from build123d import *

# Parameters (mm, degrees)
BOSS_EXTRUDE6_DEPTH      = 22.6
BOSS_EXTRUDE6_DEPTH_BACK = 22.6
SKETCH9_R                = 1.5
BOSS_EXTRUDE7_START      = -22.6
BOSS_EXTRUDE7_OUTLINE_R  = 2.5
BOSS_EXTRUDE7_DEPTH      = 45.2
CUT_EXTRUDE1_DEPTH       = 21.2
CUT_EXTRUDE1_DEPTH_BACK  = 21.2
SKETCH9_30_R             = 1.5
BOSS_EXTRUDE8_DEPTH      = 22.6
BOSS_EXTRUDE8_DEPTH_BACK = 22.6
SKETCH9_31_R             = 1.5
FILLET1_R                = 4
CHAMFER1_SIZE            = 2
CHAMFER2_SIZE            = 10
SKETCH11_R               = 2.5
CUT_EXTRUDE5_DEPTH       = 4


# Read off the part's stored shape, not the designer's step: Boss-Extrude7
with BuildPart() as part:
    # Sketch9 → Boss-Extrude6 (new, two sides: drawn at the far end of the back side and taken through both)
    with BuildSketch(Plane.XY.offset(-BOSS_EXTRUDE6_DEPTH_BACK)):
        Polygon((10.55, -1.2), (30.962513099, -1.2), (30.962513099, 6.2), (25.90954056, 6.2), (25.90954056, 8.2), (25.90954056, 18), (9.45, 18), (7.014466094, 15.564466094), (7.014466094, 11.55), (10.55, 8.014466094), align=None)
        with Locations((15.35, 2.8)):
            Circle(SKETCH9_R, mode=Mode.SUBTRACT)
    extrude(amount=BOSS_EXTRUDE6_DEPTH + BOSS_EXTRUDE6_DEPTH_BACK)

    # Boss-Extrude7 outline → Boss-Extrude7 (add)
    with BuildSketch(Plane.XY.offset(BOSS_EXTRUDE7_START)):
        with BuildLine():
            Line((38.90954056, 18), (25.90954056, 18))
            Line((25.90954056, 18), (25.90954056, 16))
            Line((25.90954056, 16), (38.90954056, 16))
            ThreePointArc((38.90954056, 16), (67.193811807, 4.284271247), (78.90954056, -24))
            Line((78.90954056, -24), (78.90954056, -78))
            ThreePointArc((78.90954056, -78), (71.880103308, -94.970562748), (54.90954056, -102))
            Line((54.90954056, -102), (54.709540559, -102))
            ThreePointArc((54.709540559, -102), (37.738977811, -94.970562748), (30.709540559, -78))
            Line((30.709540559, -78), (30.709540559, -24.386722193))
            ThreePointArc((30.709540559, -24.386722193), (37.738977811, -7.416159445), (54.709540559, -0.386722193))
            Line((54.709540559, -0.386722193), (57.736465726, -0.386722193))
            ThreePointArc((57.736465726, -0.386722193), (61.526284336, -3.986931746), (64.638517317, -8.186722193))
            Line((64.638517317, -8.186722193), (54.709540559, -8.186722193))
            ThreePointArc((54.709540559, -8.186722193), (43.254410704, -12.931592338), (38.509540559, -24.386722193))
            Line((38.509540559, -24.386722193), (38.509540559, -78))
            ThreePointArc((38.509540559, -78), (43.254410704, -89.455129855), (54.709540559, -94.2))
            Line((54.709540559, -94.2), (54.90954056, -94.2))
            ThreePointArc((54.90954056, -94.2), (66.364670415, -89.455129855), (71.10954056, -78))
            Line((71.10954056, -78), (71.10954056, -24))
            ThreePointArc((71.10954056, -24), (61.678378914, -1.231161646), (38.90954056, 8.2))
            Line((38.90954056, 8.2), (25.90954056, 8.2))
            Line((25.90954056, 8.2), (25.90954056, 6.2))
            Line((25.90954056, 6.2), (30.962513099, 6.2))
            Line((30.962513099, 6.2), (30.962513099, -13.8))
            ThreePointArc((30.962513099, -13.8), (29.279020372, -18.974823911), (28.709540559, -24.386722193))
            Line((28.709540559, -24.386722193), (28.709540559, -78))
            ThreePointArc((28.709540559, -78), (36.324764249, -96.384776311), (54.709540559, -104))
            Line((54.709540559, -104), (54.90954056, -104))
            ThreePointArc((54.90954056, -104), (73.29431687, -96.384776311), (80.90954056, -78))
            Line((80.90954056, -78), (80.90954056, -24))
            ThreePointArc((80.90954056, -24), (68.608025369, 5.69848481), (38.90954056, 18))
        make_face()
        with BuildLine():
            Line((40.509540559, -78), (40.509540559, -52.193361097))
            Line((40.509540559, -52.193361097), (48.38692427, -52.193361097))
            ThreePointArc((48.38692427, -52.193361097), (50.213346482, -55.789555174), (53.809540559, -57.615977386))
            Line((53.809540559, -57.615977386), (53.809540559, -92.171450173))
            ThreePointArc((53.809540559, -92.171450173), (44.355314369, -87.717509969), (40.509540559, -78))
        make_face(mode=Mode.SUBTRACT)
        with BuildLine():
            Line((61.232156849, -52.193361097), (69.10954056, -52.193361097))
            Line((69.10954056, -52.193361097), (69.10954056, -78))
            ThreePointArc((69.10954056, -78), (65.26376675, -87.717509969), (55.80954056, -92.171450173))
            Line((55.80954056, -92.171450173), (55.809540559, -57.615977386))
            ThreePointArc((55.809540559, -57.615977386), (59.405734637, -55.789555174), (61.232156849, -52.193361097))
        make_face(mode=Mode.SUBTRACT)
        with Locations((54.809540559, -51.193361097)):
            Circle(BOSS_EXTRUDE7_OUTLINE_R, mode=Mode.SUBTRACT)
        with BuildLine():
            Line((48.38692427, -50.193361097), (40.509540559, -50.193361097))
            Line((40.509540559, -50.193361097), (40.509540559, -24.386722193))
            ThreePointArc((40.509540559, -24.386722193), (44.321085429, -14.705813145), (53.709540559, -10.221977225))
            Line((53.709540559, -10.221977225), (53.709540559, -44.787114146))
            ThreePointArc((53.709540559, -44.787114146), (50.177660219, -46.633132538), (48.38692427, -50.193361097))
        make_face(mode=Mode.SUBTRACT)
        with BuildLine():
            ThreePointArc((38.90954056, 6.2), (47.231770136, 5.030681957), (54.909540559, 1.613277807))
            Line((54.909540559, 1.613277807), (54.709540559, 1.613277807))
            ThreePointArc((54.709540559, 1.613277807), (43.121398237, -1.111951356), (33.962513099, -8.716340846))
            Line((33.962513099, -8.716340846), (33.962513099, 6.2))
            Line((33.962513099, 6.2), (38.90954056, 6.2))
        make_face(mode=Mode.SUBTRACT)
        with BuildLine():
            Line((55.709540559, -10.186722193), (65.765328692, -10.186722193))
            ThreePointArc((65.765328692, -10.186722193), (68.261583092, -16.89383372), (69.10954056, -24))
            Line((69.10954056, -24), (69.10954056, -50.193361097))
            Line((69.10954056, -50.193361097), (61.232156849, -50.193361097))
            ThreePointArc((61.232156849, -50.193361097), (59.369856551, -46.561566838), (55.709540559, -44.755970321))
            Line((55.709540559, -44.755970321), (55.709540559, -10.186722193))
        make_face(mode=Mode.SUBTRACT)
    extrude(amount=BOSS_EXTRUDE7_DEPTH)

    # Sketch9<30> → Cut-Extrude1 (cut, two sides: drawn at the far end of the back side and taken through both)
    # profile 1 of 2: a face of its own
    with BuildSketch(Plane.XY.offset(-CUT_EXTRUDE1_DEPTH_BACK)):
        Polygon((19.104002376, 5), (16.104002376, 5), (10.55, 4), (10.55, -1.2), (19.35, -1.2), (19.35, 5.043376018), align=None)
        with Locations((15.35, 2.8)):
            Circle(SKETCH9_30_R, mode=Mode.SUBTRACT)
    # profile 2 of 2: a face of its own
    with BuildSketch(Plane.XY.offset(-CUT_EXTRUDE1_DEPTH_BACK)):
        Polygon((10.55, 5.097056275), (16.104002376, 7), (19.104002376, 7), (25.90954056, 8.2), (25.90954056, 16), (16.104002376, 16), (7.014466094, 14.164466094), (7.014466094, 11.55), (10.55, 8.014466094), align=None)
    extrude(amount=CUT_EXTRUDE1_DEPTH + CUT_EXTRUDE1_DEPTH_BACK, mode=Mode.SUBTRACT)

    # Sketch9<31> → Boss-Extrude8 (add, two sides: drawn at the far end of the back side and taken through both)
    # profile 1 of 2: a face of its own
    with BuildSketch(Plane.XY.offset(-BOSS_EXTRUDE8_DEPTH_BACK)):
        with BuildLine():
            ThreePointArc((38.90954056, 18), (56.770808698, 14.012828104), (71.240841297, 2.808338118))
            Line((71.240841297, 2.808338118), (71.240841297, 8))
            Line((71.240841297, 8), (71.240841297, 18))
            Line((71.240841297, 18), (38.90954056, 18))
        make_face()
        with Locations((66.240841297, 13)):
            Circle(SKETCH9_31_R, mode=Mode.SUBTRACT)
    # profile 2 of 2: a face of its own
    with BuildSketch(Plane.XY.offset(-BOSS_EXTRUDE8_DEPTH_BACK)):
        with BuildLine():
            Line((54.709540559, -104), (54.90954056, -104))
            ThreePointArc((54.90954056, -104), (57.370590519, -103.88326164), (59.809540559, -103.534094854))
            Line((59.809540559, -103.534094854), (59.809540559, -112))
            Line((59.809540559, -112), (49.809540559, -112))
            Line((49.809540559, -112), (49.809540559, -103.534094854))
            ThreePointArc((49.809540559, -103.534094854), (52.2484906, -103.88326164), (54.709540559, -104))
        make_face()
        with Locations((54.809540559, -108)):
            Circle(SKETCH9_31_R, mode=Mode.SUBTRACT)
    extrude(amount=BOSS_EXTRUDE8_DEPTH + BOSS_EXTRUDE8_DEPTH_BACK)

    # Fillet1
    fillet1_edges = [part.edges().sort_by_distance(p)[0] for p in [
        (71.240841297, 18, 0),
        (59.809540559, -112, 0),
        (49.809540559, -112, 0),
    ]]
    fillet(fillet1_edges, radius=FILLET1_R)

    # Chamfer1
    chamfer1_edges = [part.edges().sort_by_distance(p)[0] for p in [
        (10.55, -1.2, -21.9),
        (10.55, -1.2, 21.9),
    ]]
    chamfer(chamfer1_edges, length=CHAMFER1_SIZE)

    # Chamfer2
    # the kernel refuses this chamfer: 10 mm, written as the material it adds along each edge
    with BuildSketch(Plane(origin=(19.35, -1.2, -21.2), x_dir=(0.027495876610586317, 0, 0.9996219169112968), z_dir=(0, 1, 0))) as chamfer2_piece_1_section:
        Polygon((CHAMFER2_SIZE * 0.999621916911, -CHAMFER2_SIZE * 0.0274958766106), (-CHAMFER2_SIZE * 0.0274958766106, -CHAMFER2_SIZE * 0.999621916911), (0, 0), align=None)
    chamfer2_piece_1 = extrude(amount=31.960205898, mode=Mode.PRIVATE)
    chamfer2_piece_1 = split(chamfer2_piece_1, bisect_by=Plane(origin=(10.55, 0.553309939, -18.301201582), z_dir=(1, 0, 0)), keep=Keep.TOP, mode=Mode.PRIVATE)
    chamfer2_piece_1 = split(chamfer2_piece_1, bisect_by=Plane(origin=(12.972143449, -1.622143449, -18.301201582), z_dir=(0.707106781186546, 0.7071067811865491, 0)), keep=Keep.TOP, mode=Mode.PRIVATE)
    chamfer2_piece_1 = split(chamfer2_piece_1, bisect_by=Plane(origin=(13.271329508, 6.029453592, -18.301201582), z_dir=(0.32412836516113813, -0.9460131092632744, 0)), keep=Keep.TOP, mode=Mode.PRIVATE)
    chamfer2_piece_1 = chamfer2_piece_1 - Plane(origin=(15.35, 2.8, -18.301201582), x_dir=(1, 0, 0), z_dir=(0, 0, -1)) * Cylinder(1.5, 104, mode=Mode.PRIVATE)
    chamfer2_piece_1 = split(chamfer2_piece_1, bisect_by=Plane(origin=(15.147596837, 7, -18.301201582), z_dir=(0, -1, 0)), keep=Keep.TOP, mode=Mode.PRIVATE)
    add(chamfer2_piece_1)
    with BuildSketch(Plane(origin=(19.35, -1.2, 21.2), x_dir=(-0.9996219169112968, 0, 0.027495876610586317), z_dir=(0, 1, 0))) as chamfer2_piece_2_section:
        Polygon((CHAMFER2_SIZE * 0.999621916911, -CHAMFER2_SIZE * 0.0274958766106), (-CHAMFER2_SIZE * 0.0274958766106, -CHAMFER2_SIZE * 0.999621916911), (0, 0), align=None)
    chamfer2_piece_2 = extrude(amount=31.960205898, mode=Mode.PRIVATE)
    chamfer2_piece_2 = split(chamfer2_piece_2, bisect_by=Plane(origin=(12.972143449, -1.622143449, 18.301201581), z_dir=(0.707106781186546, 0.7071067811865491, 0)), keep=Keep.TOP, mode=Mode.PRIVATE)
    chamfer2_piece_2 = split(chamfer2_piece_2, bisect_by=Plane(origin=(10.55, 0.553309939, 18.301201581), z_dir=(1, 0, 0)), keep=Keep.TOP, mode=Mode.PRIVATE)
    chamfer2_piece_2 = chamfer2_piece_2 - Plane(origin=(15.35, 2.8, 18.301201581), x_dir=(1, 0, 0), z_dir=(0, 0, -1)) * Cylinder(1.5, 104, mode=Mode.PRIVATE)
    chamfer2_piece_2 = split(chamfer2_piece_2, bisect_by=Plane(origin=(13.271329509, 6.029453592, 18.301201581), z_dir=(0.32412836516113813, -0.9460131092632744, 0)), keep=Keep.TOP, mode=Mode.PRIVATE)
    chamfer2_piece_2 = split(chamfer2_piece_2, bisect_by=Plane(origin=(15.147596837, 7, 18.301201581), z_dir=(0, -1, 0)), keep=Keep.TOP, mode=Mode.PRIVATE)
    add(chamfer2_piece_2)

    # Sketch11 → Cut-Extrude5 (cut)
    with BuildSketch(Plane.XZ.offset(1.2)):
        with Locations(Location((23.35, 10, 0), (0, 0, 270))):
            Circle(SKETCH11_R)
        with Locations(Location((23.35, -10, 0), (0, 0, 270))):
            Circle(SKETCH11_R)
    extrude(amount=-CUT_EXTRUDE5_DEPTH, mode=Mode.SUBTRACT)


solid = part.part
Model file for the job. Use its own axes, mm. A direction names the side the tool comes from. Give positions to 0.01 mm unless a question says otherwise; leave off trailing zeros. Loops run counter-clockwise (first coordinate to the right, second up) from the corner with the lowest first, then second, coordinate; pieces in that order, holes last. Notation, with made-up numbers: (71, -26) -> (91, -26) arc R24 ccw to (91, -5) -> close; hole circle Ø6 at (8, -9). An arc over 180 degrees is marked (long way). Use a Markdown table: item, result. Add a question column.
(1) Slice it at B-B on x = 23.35. List the corners of the cut face in (y, z).
(2) Mould opens along Y. For faces 1 (the flat face through (56, -0.387, 0)), 2 (the flat face through (8.757, 9.807, -21.91)), 3 (the cylindrical face through (59.41, -46.6, -0.32)), 4 (the cylindrical face through (70.04, 16.86, 0.32)) say: +Y half, -Y half, draft (parallel to the pull), parting line (faces both ways), or undercut.
(3) Slice it at D-D on y = -82. List the corners of the cut face in (x, z), and give its area (3 significant figures).
(4) Slice it at C-C on x = 45. List the corners of the cut face in (y, z).
(5) Slice it at A-A on y = -36. List the corners of the cut face in (x, z), and give its area (3 significant figures).
(6) Drop flat-ended pins along their axis: pin 1 Ø1.5 at (x, z) = (37, -4.5) entering from -Y; pin 2 Ø10.5 at (y, z) = (-72, 5) entering from -X; pin 3 Ø0.9 at (x, z) = (56.5, -11) entering from -Y. Give the stop position or say it passes through.
(7) Wall check: line 1 along Y through (x, z) = (17, -18.5); line 2 along X through (y, z) = (-68.5, -19.5); line 3 along X through (y, z) = (-108, 3.5). Give the ranges that are in metal, low to high.
(8) Tool access for faces 5 (the flat face through (23, 2.8, 10)), 6 (the flat face through (18, 7, 0)), 7 (the flat face through (36, 6.2, 0)), 8 (the cylindrical face through (29.295, -18.9, -0.316)): list every direction of +Z, -Z, +X, -X, +Y, -Y with a clear straight run to the whole face (end or side of a thin tool).
Filled sheet:
| question | item | result |
|---|---|---|
| 1 | outline | (-1.2, -22.6) -> (18, -22.6) -> (18, 22.6) -> (-1.2, 22.6) -> (-1.2, 12.5) -> (2.8, 12.5) -> (2.8, 7.5) -> (-1.2, 7.5) -> (-1.2, -7.5) -> (2.8, -7.5) -> (2.8, -12.5) -> (-1.2, -12.5) -> close; hole (7.75, -21.2) -> (16, -21.2) -> (16, 21.2) -> (7.75, 21.2) -> close |
| 2 | face 1 | undercut |
| 2 | face 2 | -Y half |
| 2 | face 3 | undercut |
| 2 | face 4 | +Y half |
| 3 | outline | (29.02, -22.6) -> (31.05, -22.6) -> (31.05, 22.6) -> (29.02, 22.6) -> close; (39.01, -22.6) -> (41.08, -22.6) -> (41.08, 22.6) -> (39.01, 22.6) -> close; (53.81, -22.6) -> (55.81, -22.6) -> (55.81, 22.6) -> (53.81, 22.6) -> close; (68.53, -22.6) -> (70.61, -22.6) -> (70.61, 22.6) -> (68.53, 22.6) -> close; (78.57, -22.6) -> (80.6, -22.6) -> (80.6, 22.6) -> (78.57, 22.6) -> close |
| 3 | area | 461 mm2 |
| 4 | outline | (-102.12, -22.6) -> (-99.95, -22.6) -> (-99.95, 22.6) -> (-102.12, 22.6) -> close; (-90.97, -22.6) -> (-88.36, -22.6) -> (-88.36, 22.6) -> (-90.97, 22.6) -> close; (-52.19, -22.6) -> (-50.19, -22.6) -> (-50.19, 22.6) -> (-52.19, 22.6) -> close; (-14.03, -22.6) -> (-11.42, -22.6) -> (-11.42, 22.6) -> (-14.03, 22.6) -> close; (-2.44, -22.6) -> (-0.27, -22.6) -> (-0.27, 22.6) -> (-2.44, 22.6) -> close; (5.58, -22.6) -> (7.62, -22.6) -> (7.62, 22.6) -> (5.58, 22.6) -> close; (15.53, -22.6) -> (18, -22.6) -> (18, 22.6) -> (15.53, 22.6) -> close |
| 5 | outline | (28.71, -22.6) -> (30.71, -22.6) -> (30.71, 22.6) -> (28.71, 22.6) -> close; (38.51, -22.6) -> (40.51, -22.6) -> (40.51, 22.6) -> (38.51, 22.6) -> close; (53.71, -22.6) -> (55.71, -22.6) -> (55.71, 22.6) -> (53.71, 22.6) -> close; (69.11, -22.6) -> (71.11, -22.6) -> (71.11, 22.6) -> (69.11, 22.6) -> close; (78.91, -22.6) -> (80.91, -22.6) -> (80.91, 22.6) -> (78.91, 22.6) -> close |
| 5 | area | 452 mm2 |
| 6 | pin 1 | y = -97.71 |
| 6 | pin 2 | x = 28.71 |
| 6 | pin 3 | y = -111.99 |
| 7 | line 1 | -1.2 to 7, 16 to 18 |
| 7 | line 2 | 28.71 to 30.71, 38.51 to 40.51, 53.81 to 55.81, 69.11 to 71.11, 78.91 to 80.91 |
| 7 | line 3 | 49.81 to 53.31, 56.31 to 59.81 |
| 8 | face 5 | -Y |
| 8 | face 6 | -X |
| 8 | face 7 | +Z, -Z |
| 8 | face 8 | +Z, -Z, -X |
